Geometry: final body of the model. Coordinates: model frame, mm. A direction names the side the tool comes from. Give positions to 0.01 mm unless a question says otherwise; leave off trailing zeros. Write each loop counter-clockwise with the first axis right and the second up, starting at its lowest first coordinate (ties: lowest second). Pieces come first, ordered by that corner, then holes. Notation, with made-up numbers: (5, 72) -> (32, 72) arc R22 cw to (32, 84) -> close; hole circle Ø1 at (7, 62.5). An arc over 180 degrees is marked (long way). Answer as a JSON object with one key per item and string values.
from build123d import *

# Parameters (mm, degrees)
F0_W     = 42.3
F0_H     = 42.3
F0_R     = 1.65
F0_R_2   = 13
F1_DEPTH = 4
F2_R     = 5
F4_DEPTH = 38.36
F5_W     = 42.3
F5_H     = 42.200226
F5_R     = 1.65
F5_R_2   = 13
F6_DEPTH = 4
F7_R     = 5


with BuildPart() as f1:
    # F0 (on Top) → F1 (new body)
    with BuildSketch(Plane.XY):
        Rectangle(F0_W, F0_H)
        with Locations((-15.5, -15.5)):
            Circle(F0_R, mode=Mode.SUBTRACT)
        with Locations((15.5, -15.5)):
            Circle(F0_R, mode=Mode.SUBTRACT)
        with Locations((-15.5, 15.5)):
            Circle(F0_R, mode=Mode.SUBTRACT)
        Circle(F0_R_2, mode=Mode.SUBTRACT)
        with Locations((15.5, 15.5)):
            Circle(F0_R, mode=Mode.SUBTRACT)
    extrude(amount=F1_DEPTH)

    # F2
    f2_edges = [f1.edges().sort_by_distance(p)[0] for p in [
        (-21.15, -21.15, 2),
        (21.15, -21.15, 2),
        (-21.15, 21.15, 2),
        (21.15, 21.15, 2),
    ]]
    fillet(f2_edges, radius=F2_R)

    # F3 (on face) → F4 (join)
    with BuildSketch(Plane.XY.offset(4)):
        with BuildLine():
            ThreePointArc((-15.5, 9.812734), (-17.633029, 10.227886), (-19.454649, 11.412733))
            ThreePointArc((-19.454649, 11.412733), (-20.540287, 11.614756), (-21.15, 10.694063))
            Line((-21.15, 10.694063), (-21.15, -10.746054))
            ThreePointArc((-21.15, -10.746054), (-20.537783, -11.667805), (-19.450752, -11.460933))
            ThreePointArc((-19.450752, -11.460933), (-17.633281, -10.268211), (-15.5, -9.85))
            Line((-15.5, -9.85), (-15.5, 9.812734))
        make_face()
        with BuildLine():
            ThreePointArc((9.812734, 15.5), (10.227886, 17.633029), (11.412733, 19.454649))
            ThreePointArc((11.412733, 19.454649), (11.614756, 20.540287), (10.694063, 21.15))
            Line((10.694063, 21.15), (-10.694063, 21.15))
            ThreePointArc((-10.694063, 21.15), (-11.614756, 20.540287), (-11.412733, 19.454649))
            ThreePointArc((-11.412733, 19.454649), (-10.227886, 17.633029), (-9.812734, 15.5))
            Line((-9.812734, 15.5), (9.812734, 15.5))
        make_face()
        with BuildLine():
            ThreePointArc((15.5, -9.812734), (17.633029, -10.227886), (19.454649, -11.412733))
            ThreePointArc((19.454649, -11.412733), (20.540287, -11.614756), (21.15, -10.694063))
            Line((21.15, -10.694063), (21.15, 10.694063))
            ThreePointArc((21.15, 10.694063), (20.540287, 11.614756), (19.454649, 11.412733))
            ThreePointArc((19.454649, 11.412733), (17.633029, 10.227886), (15.5, 9.812734))
            Line((15.5, 9.812734), (15.5, -9.812734))
        make_face()
    extrude(amount=F4_DEPTH)

    # F5 (on face) → F6 (join)
    with BuildSketch(Plane.XY.offset(42.36)):
        Rectangle(F5_W, F5_H)
        with Locations((-15.5, -15.5)):
            Circle(F5_R, mode=Mode.SUBTRACT)
        with Locations((15.5, -15.5)):
            Circle(F5_R, mode=Mode.SUBTRACT)
        with Locations((-15.5, 15.5)):
            Circle(F5_R, mode=Mode.SUBTRACT)
        Circle(F5_R_2, mode=Mode.SUBTRACT)
        with Locations((15.5, 15.5)):
            Circle(F5_R, mode=Mode.SUBTRACT)
    extrude(amount=F6_DEPTH)

    # F7
    f7_edges = [f1.edges().sort_by_distance(p)[0] for p in [
        (-21.15, -21.100113, 44.36),
        (21.15, -21.100113, 44.36),
        (-21.15, 21.100113, 44.36),
        (21.15, 21.100113, 44.36),
    ]]
    fillet(f7_edges, radius=F7_R)


solid = f1.part
Q1. Cut plane C-C (x = 0). Return the cut outline in (y, z).
Values:
{"outline": "(-21.15, 0) -> (-13, 0) -> (-13, 4) -> (-21.15, 4) -> close; (-21.1, 42.36) -> (-13, 42.36) -> (-13, 46.36) -> (-21.1, 46.36) -> close; (13, 0) -> (21.15, 0) -> (21.15, 42.36) -> (21.1, 42.36) -> (21.1, 46.36) -> (13, 46.36) -> (13, 42.36) -> (15.5, 42.36) -> (15.5, 4) -> (13, 4) -> close"}
Q2. Cut plane D-D (x = 14.5). Return the cut outline in (y, z), and give its area (3 significant figures).
Values:
{"outline": "(-21.15, 0) -> (-16.81, 0) -> (-16.81, 4) -> (-21.15, 4) -> close; (-21.1, 42.36) -> (-16.81, 42.36) -> (-16.81, 46.36) -> (-21.1, 46.36) -> close; (-14.19, 0) -> (14.19, 0) -> (14.19, 4) -> (-14.19, 4) -> close; (-14.19, 42.36) -> (14.19, 42.36) -> (14.19, 46.36) -> (-14.19, 46.36) -> close; (16.81, 0) -> (21.15, 0) -> (21.15, 4) -> (16.81, 4) -> close; (16.81, 42.36) -> (21.1, 42.36) -> (21.1, 46.36) -> (16.81, 46.36) -> close", "area": "296 mm²"}
Q3. Cut plane A-A (y = 0). Return the cut outline in (x, z).
Values:
{"outline": "(-21.15, 0) -> (-13, 0) -> (-13, 4) -> (-15.5, 4) -> (-15.5, 42.36) -> (-13, 42.36) -> (-13, 46.36) -> (-21.15, 46.36) -> close; (13, 0) -> (21.15, 0) -> (21.15, 46.36) -> (13, 46.36) -> (13, 42.36) -> (15.5, 42.36) -> (15.5, 4) -> (13, 4) -> close"}
Q4. Mould query, pull axis Z, two halves, no side actions, for faces 1 (the cylindrical face through (-10.316, -7.91, 44.332)), 2 (the flat face through (0, -14, 4)). Classes: pulls with the +Z half, pulls with the -Z half, needs draft (parallel to the pull), parting line crosses it, or undercut.
Values:
{"face 1": "needs draft", "face 2": "undercut"}
Q5. Set-up query: faces 3 (the cylindrical face through (10.216, 17.605, 22.911)), 4 (the flat face through (0, -21.1, 44)), 5 (the cylindrical face through (17.605, -10.216, 22.911)), 6 (the cylindrical face through (-19.72, -19.6, 44.39)), 7 (the cylindrical face through (17.66, 10.24, 22.91)). Return all of +Z, -Z, +X, -X, +Y, -Y with unobstructed straight access to the full face (end or side cutting, diameter ignored); none if empty.
Values:
{"face 3": "+X, -Y", "face 4": "+Z, +X, -X, -Y", "face 5": "-Y", "face 6": "+Z, -X, -Y", "face 7": "+Y"}
Q6. Cut plane B-B (z = 19.5). Return the cut outline in (x, y), and give its area (3 significant figures).
Values:
{"outline": "(-21.15, -10.75) arc R1 ccw to (-19.45, -11.46) arc R5.65 cw to (-15.5, -9.85) -> (-15.5, 9.81) arc R5.69 cw to (-19.45, 11.41) arc R1 ccw to (-21.15, 10.69) -> close; (-11.41, 19.45) arc R5.69 cw to (-9.81, 15.5) -> (9.81, 15.5) arc R5.69 cw to (11.41, 19.45) arc R1 ccw to (10.69, 21.15) -> (-10.69, 21.15) arc R1 ccw to start; (15.5, -9.81) arc R5.69 cw to (19.45, -11.41) arc R1 ccw to (21.15, -10.69) -> (21.15, 10.69) arc R1 ccw to (19.45, 11.41) arc R5.69 cw to (15.5, 9.81) -> close", "area": "362 mm²"}
Q7. First-contact query: P1, Ø6, axis at y = 16, z = 22, coming from the -X side; P2, Ø8, axis at x = -4.5, z = 21, coming from the -Y side; P3, Ø1.2, axis at x = -3, z = 45, coming from the -Y side. Flat tips, straight axial feed; report the tip coordinate or a pass-through.
Values:
{"P1": "x = -11.02", "P2": "y = 15.5", "P3": "y = -21.1"}
Q8. Material intervals for L1, parallel to Y at x = 15.5, z = 2.6; L2, parallel to Z at x = 10.5, y = -14; L3, parallel to X at y = 4.5, z = 23.5, sorted ascending. Write a range as from..to.
Values:
{"L1": "-21.15..-17.15, -13.85..13.85, 17.15..21.15", "L2": "0..4, 42.36..46.36", "L3": "-21.15..-15.5, 15.5..21.15"}
